Here's how the part is built. I have some questions about the finished solid (model axes, mm). A direction names the side the tool comes from. Coordinates: 2 decimals unless noted, no trailing zeros. Order: outer loops, then holes, each group sorted by start corner. A loop starts at its lowest first (then second) coordinate and runs counter-clockwise, first axis right, second up. Notation, with made-up numbers: (-32, -36.5) - (23, -36.5) arc R19 ccw to (23, -20.5) - close; hole circle Ø6 at (-1, 16.25). An arc over 180 degrees is marked (long way). Answer as CSV lines item,"result". Start each with the question number.
Q1. For pin 1 Ø1.1 at (y, z) = (16, 0.5) entering from -X; pin 2 Ø0.8 at (y, z) = (16.5, 0.5) entering from +X; pin 3 Ø1.1 at (y, z) = (-17, 0.5) entering from +X; pin 4 Ø1 at (x, y) = (-9, 11.5) entering from -Z, each with a flat end and sliding along its axis, tell me the tip position at first contact or that it passes through.
Q2. Suppose I cut it at A-A (x = 0). Please give me the cut outline in (y, z) (3 decimals).
Q3. I need wall thicknesses on line 1 (X direction, y = 0, z = 3) (3 decimals); line 2 (Y direction, x = 11, z = 2). Which ranges of each line are inside material? Lowest first, please.
Q4. Suppose I cut it at B-B (y = 0). Please give me the cut outline in (x, z) (3 decimals).
Q5. Suppose I cut it at C-C (z = 3.5). Please give me the cut outline in (x, y) (1 decimal), then the cut area to 3 significant figures.
Q6. Suppose I cut it at D-D (y = 6). Please give me the cut outline in (x, z) (3 decimals), then the cut area to 3 significant figures.
Q7. For faces 1 (the face through (-6.987, -0.214, 4.686)), 2 (the face through (-6.414, 16.3, 0.5)), 3 (the face through (-7.6, 17.78, 0.5)), 4 (the face through (9.716, 17, 5)), 5 (the face through (-16.4, 6.414, 0.5)), which set-ups out of +Z, -Z, +X, -X, +Y, -Y let a thin tool reach every point of the face, with its end or its side?
from build123d import *

# Parameters (mm, degrees)
F1_DEPTH = 8.255
F3_DEPTH = 7.239
F5_DEPTH = 25.4
F6_R     = 8.89
F7_R     = 4.445
F8_DEPTH = 25.4


with BuildPart() as f1:
    # F0 (on Top) → F1 (new body)
    with BuildSketch(Plane.XY):
        Polygon((8.144473, -17.78), (17.78, -17.78), (17.78, 17.78), (-17.78, 17.78), (-17.78, -17.78), (-8.144473, -17.78), align=None)
    extrude(amount=F1_DEPTH)

    # F2 (on face) → F3 (cut)
    with BuildSketch(Plane.XY.offset(8.255)):
        with BuildLine():
            Line((-9.7155, 17.78), (-9.7155, 16.7005))
            ThreePointArc((-9.7155, 16.7005), (0, 6.985), (9.7155, 16.7005))
            Line((9.7155, 16.7005), (9.7155, 17.78))
            Line((9.7155, 17.78), (-9.7155, 17.78))
        make_face()
        with BuildLine():
            Line((17.78, 9.7155), (16.7005, 9.7155))
            ThreePointArc((16.7005, 9.7155), (6.985, 0), (16.7005, -9.7155))
            Line((16.7005, -9.7155), (17.78, -9.7155))
            Line((17.78, -9.7155), (17.78, 9.7155))
        make_face()
        with BuildLine():
            Line((-17.78, -9.7155), (-16.7005, -9.7155))
            ThreePointArc((-16.7005, -9.7155), (-6.985, 0), (-16.7005, 9.7155))
            Line((-16.7005, 9.7155), (-17.78, 9.7155))
            Line((-17.78, 9.7155), (-17.78, -9.7155))
        make_face()
        with BuildLine():
            Line((9.7155, -17.78), (9.7155, -16.7005))
            ThreePointArc((9.7155, -16.7005), (0, -6.985), (-9.7155, -16.7005))
            Line((-9.7155, -16.7005), (-9.7155, -17.78))
            Line((-9.7155, -17.78), (9.7155, -17.78))
        make_face()
    extrude(amount=-F3_DEPTH, mode=Mode.SUBTRACT)

    # F4 (on face) → F5 (cut)
    with BuildSketch(Plane(origin=(0, 0, 0), x_dir=(1, 0, 0), z_dir=(0, 0, -1))):
        with BuildLine():
            Line((-6.4135, 17.78), (-6.4135, 15.3035))
            ThreePointArc((-6.4135, 15.3035), (0, 8.89), (6.4135, 15.3035))
            Line((6.4135, 15.3035), (6.4135, 17.78))
            Line((6.4135, 17.78), (-6.4135, 17.78))
        make_face()
        with BuildLine():
            Line((17.78, 6.4135), (14.5415, 6.4135))
            ThreePointArc((14.5415, 6.4135), (8.128, 0), (14.5415, -6.4135))
            Line((14.5415, -6.4135), (17.78, -6.4135))
            Line((17.78, -6.4135), (17.78, 6.4135))
        make_face()
        with BuildLine():
            Line((-17.78, -6.4135), (-15.0495, -6.4135))
            ThreePointArc((-15.0495, -6.4135), (-8.636, 0), (-15.0495, 6.4135))
            Line((-15.0495, 6.4135), (-17.78, 6.4135))
            Line((-17.78, 6.4135), (-17.78, -6.4135))
        make_face()
        with BuildLine():
            Line((6.4135, -17.78), (6.4135, -14.7955))
            ThreePointArc((6.4135, -14.7955), (0, -8.382), (-6.4135, -14.7955))
            Line((-6.4135, -14.7955), (-6.4135, -17.78))
            Line((-6.4135, -17.78), (6.4135, -17.78))
        make_face()
    extrude(amount=-F5_DEPTH, mode=Mode.SUBTRACT)

    # F6
    f6_edges = [f1.edges().sort_by_distance(p)[0] for p in [
        (-17.78, 17.78, 4.1275),
        (-17.78, -17.78, 4.1275),
        (17.78, -17.78, 4.1275),
        (17.78, 17.78, 4.1275),
    ]]
    fillet(f6_edges, radius=F6_R)

    # F7 (on face) → F8 (cut)
    with BuildSketch(Plane(origin=(0, 0, 0), x_dir=(1, 0, 0), z_dir=(0, 0, -1))):
        Circle(F7_R)
    extrude(amount=-F8_DEPTH, mode=Mode.SUBTRACT)


solid = f1.part
Here are the results:
1,pin 1,"stops at x = -14.89"
1,pin 2,"stops at x = 14.09"
1,pin 3,"stops at x = 13.57"
1,pin 4,"stops at z = 0"
2,outline,"(-8.89, 0) - (-4.445, 0) - (-4.445, 8.255) - (-6.985, 8.255) - (-6.985, 1.016) - (-8.89, 1.016) - close; (4.445, 0) - (8.382, 0) - (8.382, 1.016) - (6.985, 1.016) - (6.985, 8.255) - (4.445, 8.255) - close"
3,line 1,"x = -6.985 to -4.445, 4.445 to 6.985"
3,line 2,"y = -17.53 to -7.87, 7.87 to 17.53"
4,outline,"(-8.636, 0) - (-4.445, 0) - (-4.445, 8.255) - (-6.985, 8.255) - (-6.985, 1.016) - (-8.636, 1.016) - close; (4.445, 0) - (8.128, 0) - (8.128, 1.016) - (6.985, 1.016) - (6.985, 8.255) - (4.445, 8.255) - close"
5,outline,"(-17.7, -9.7) arc R8.9 ccw to (-9.7, -17.7) - (-9.7, -16.7) arc R9.7 cw to (9.7, -16.7) - (9.7, -17.7) arc R8.9 ccw to (17.7, -9.7) - (16.7, -9.7) arc R9.7 cw to (16.7, 9.7) - (17.7, 9.7) arc R8.9 ccw to (9.7, 17.7) - (9.7, 16.7) arc R9.7 cw to (-9.7, 16.7) - (-9.7, 17.7) arc R8.9 ccw to (-17.7, 9.7) - (-16.7, 9.7) arc R9.7 cw to (-16.7, -9.7) - close; hole circle Ø8.9 at (0, 0)"
5,area,"458 mm²"
6,outline,"(-12.784, 0) - (12.276, 0) - (12.276, 1.016) - (9.059, 1.016) - (9.059, 8.255) - (-9.059, 8.255) - (-9.059, 1.016) - (-12.784, 1.016) - close"
6,area,"157 mm²"
7,face 1,"+Z, -X"
7,face 2,"+Z, -Z, +Y"
7,face 3,"+Z, -Z, +X, -X, +Y"
7,face 4,"+Z, +Y"
7,face 5,"+Z, -Z, -X"
